Geometry: final body of the model. Coordinates: model frame, mm. Face numbers are marked on the shaded views. A direction names the side the tool comes from. Coordinates: 2 decimals unless noted, no trailing zeros. Loops run counter-clockwise (first coordinate to the right, second up) from the corner with the lowest first, then second, coordinate; pieces in that order, holes last. Notation, with made-up numbers: M -27,6 L -8,6 A11 ccw -8,25 Z; hole C -32.5,-6.75 d10. An arc over 180 degrees is marked long. Write item = value, one per line. Start each with the question number.
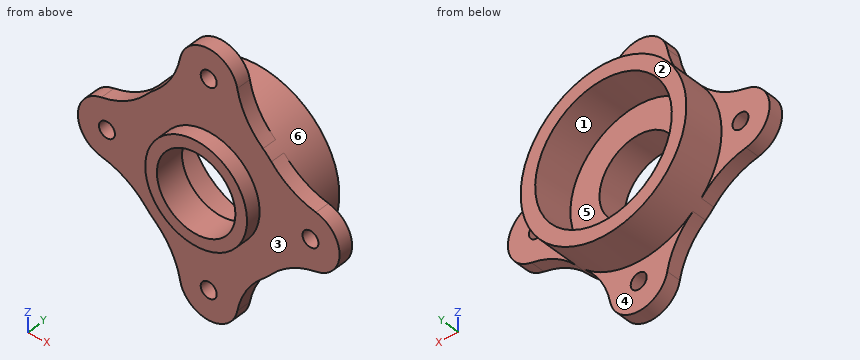
Autodesk Inventor part; units mm, degrees
ref_plane "YZ Plane" through (0, 0, 0) normal (1, 0, 0) x (0, 1, 0)
ref_plane "XZ Plane" through (0, 0, 0) normal (0, 1, 0) x (-1, 0, 0)
ref_plane "XY Plane" through (0, 0, 0) normal (0, 0, 1) x (1, 0, 0)
sketch "Sketch1" plane through (0, 0, 0) normal (1, 0, 0) x (0, 1, 0)
  line L0 (0, 0) -> (0, 23.5) construction
  line L1 (0, 23.5) -> (14, 23.5) construction
  line L2 (14, 23.5) -> (14, 0) construction
  line L3 (14, 23.5) -> (14, 28.5)
  line L4 (14, 28.5) -> (-5, 28.5)
  line L5 (14, 23.5) -> (0, 23.5)
  line L6 (-5, 28.5) -> (-5, 17.5)
  line L7 (-5, 17.5) -> (-10, 17.5)
  line L8 (-14.8, 0) -> (18.8, 0)
  line L9 (-10, 0) -> (-10, 13.5) construction
  line L10 (-10, 13.5) -> (0, 13.5)
  line L11 (0, 23.5) -> (0, 13.5)
  line L12 (-10, 17.5) -> (-10, 13.5)
  dimension "d0" = 23.5
  dimension "d1" = 14
  dimension "d2" = 5
  dimension "d3" = 19
  dimension "d8" = 11
  dimension "d9" = 5
  dimension "d11" = 13.5
revolve "Revolution1" add sketch "Sketch1" angle 360 about axis through (0, -10, 0) along (0, 1, 0)
sketch "Sketch2" plane through (0, -5, 0) normal (0, -1, 0) x (1, 0, 0)
  line L0 (-35, 0) -> (35, 0) construction
  arc A0 (-35, 10) -> (-35, -10) centre (-35, 0) ccw
  arc A1 (35, -10) -> (35, 10) centre (35, 0) ccw
  line L1 (0, -35) -> (0, 35) construction
  arc A2 (-10, -35) -> (10, -35) centre (0, -35) ccw
  arc A3 (10, 35) -> (-10, 35) centre (0, 35) ccw
  line L2 (-10, 35) -> (-10, 10)
  line L3 (-10, -10) -> (-10, -35)
  line L4 (35, 10) -> (10, 10)
  line L5 (-10, 10) -> (-35, 10)
  line L6 (10, -35) -> (10, -10)
  line L7 (10, 10) -> (10, 35)
  line L8 (-35, -10) -> (-10, -10)
  line L9 (10, -10) -> (35, -10)
  circle A4 centre (0, 0) radius 13.5
  dimension "d12" = 35
  dimension "d13" = 20
  dimension "d14" = 35
  dimension "d15" = 20
extrude "Extrusion1" add sketch "Sketch2" against normal blind 5
fillet "Fillet1" radius 27 8 edges at (10, -2.5, 26.688) (26.688, -2.5, 10) (-10, -2.5, 26.688) (-26.688, -2.5, 10) (-26.688, -2.5, -10) (-10, -2.5, -26.688) (10, -2.5, -26.688) (26.688, -2.5, -10)
hole "Hole1" at (0, -5, 35) at (35, -5, 0) at (0, -5, -35) at (-35, -5, 0) direction (0, 1, 0) diameter 5.5 end through all
properties part number "ThrustBearingMount" material "ABS Plastic"
Item 1: First-contact query: pin 1 (3 mm diameter, centred on x = -15.5, y = -0.5, fed in from -Z); pin 2 (7 mm diameter, centred on x = 0, z = -35, fed in from -Y); pin 3 (1 mm diameter, centred on x = 13.5, z = -31.5, fed in from +Y); pin 4 (7 mm diameter, centred on x = 0.5, z = -34.5, fed in from +Y). Flat tips, straight axial feed; report the tip coordinate or a pass-through.
Item 2: Section query C-C (y = -7). Return the cut outline in (x, z).
Item 3: Reachability of the marked faces 1, 2 and 3 from +Z, -Z, +X, -X, +Y, -Y: full face, straight path, thin tool, end or side. Return the list, or none.
Item 4: Section query B-B (x = 7.5). Return the cut outline in (y, z).
Item 5: Section query D-D (z = 34). Return the cut outline in (x, y), plus the area to 3 significant figures.
Item 6: Line query: line 1 (X direction, y = -2.4, z = 0); line 2 (X direction, y = 5.5, z = 1). Output: solid intervals per line, ascending. Write a range as from..to.
Item 7: Pull-direction query (X, two-part tool) for the marked faces 4, 5 and 6; classes: released by +X, released by -X, zero draft, split by the parting line, or undercut.
Item 8: Section query A-A (z = 0). Return the cut outline in (x, y), plus the area to 3 significant figures.
Verdict:
q1.pin_1 = -26.79
q1.pin_2 = -5
q1.pin_3 = through
q1.pin_4 = 0
q2.outline = C 0,0 d35; hole C 0,0 d27
q3.face_1 = +Y
q3.face_2 = +Z, -Z, +X, -X, +Y
q3.face_3 = -Y
q4.outline = M -10,-15.81 L -5,-15.81 L -5,-41.61 L 0,-41.61 L 0,-27.5 L 14,-27.5 L 14,-22.27 L 0,-22.27 L 0,-11.22 L -10,-11.22 Z; M -10,11.22 L 0,11.22 L 0,22.27 L 14,22.27 L 14,27.5 L 0,27.5 L 0,41.61 L -5,41.61 L -5,15.81 L -10,15.81 Z
q5.outline = M -10.54,-5 L -2.56,-5 L -2.56,0 L -10.54,0 Z; M 2.56,-5 L 10.54,-5 L 10.54,0 L 2.56,0 Z
q5.area = 79.8 mm2
q6.line_1 = -45..-37.75, -32.25..-13.5, 13.5..32.25, 37.75..45
q6.line_2 = -28.48..-23.48, 23.48..28.48
q7.face_4 = zero draft
q7.face_5 = undercut
q7.face_6 = split by the parting line
q8.outline = M -45,-5 L -37.75,-5 L -37.75,0 L -45,0 Z; M -32.25,-5 L -17.5,-5 L -17.5,-10 L -13.5,-10 L -13.5,0 L -23.5,0 L -23.5,14 L -28.5,14 L -28.5,0 L -32.25,0 Z; M 13.5,-10 L 17.5,-10 L 17.5,-5 L 32.25,-5 L 32.25,0 L 28.5,0 L 28.5,14 L 23.5,14 L 23.5,0 L 13.5,0 Z; M 37.75,-5 L 45,-5 L 45,0 L 37.75,0 Z
q8.area = 440 mm2
